```python
from build123d import *

# Parameters (mm, degrees)
BOSS_EXTRUDE2_DEPTH = 5


with BuildPart() as part:
    # Sketch3 → Boss-Extrude2 (new body)
    with BuildSketch(Plane(origin=(0, 0, 0), x_dir=(1, 0, 0), z_dir=(0, 1, 0))):
        with BuildLine():
            ThreePointArc((-2.946687169, 0.278195868), (-2.823196953, -0.888772849), (-2.255920315, -1.916032813))
            add(Edge.make_bspline(
                [(-2.255920315, -1.916032813), (-13.171337356, -14.504845087), (-19.982146303, -0.549733438)],
                knots=[0, 0, 0, 1, 1, 1], degree=2))
            ThreePointArc((-19.982146303, -0.549733438), (-17.317507753, -9.984603294), (-10.487312447, -17.017774689))
            add(Edge.make_bspline(
                [(-1.000187104, -2.785674778), (-2.546841566, -12.490182628), (-10.487312447, -17.017774689)],
                knots=[0, 0, 0, 1, 1, 1], degree=2))
            ThreePointArc((-1.000187104, -2.785674778), (0.084052871, -2.958596513), (1.156726663, -2.724397481))
            add(Edge.make_bspline(
                [(1.156726663, -2.724397481), (13.351165317, -11.711219241), (1.815860807, -19.907059734)],
                knots=[0, 0, 0, 1, 1, 1], degree=2))
            ThreePointArc((1.815860807, -19.907059734), (9.30002387, -17.694573568), (15.366618382, -12.784968409))
            add(Edge.make_bspline(
                [(2.913240883, -0.522863047), (17.317700847, -1.946688078), (15.366618382, -12.784968409)],
                knots=[0, 0, 0, 1, 1, 1], degree=2))
            ThreePointArc((2.913240883, -0.522863047), (2.939564994, 0.345421275), (2.712677202, 1.183951269))
            add(Edge.make_bspline(
                [(2.712677202, 1.183951269), (12.295659798, 10.008861874), (19.989706794, 0)],
                knots=[0, 0, 0, 1, 1, 1], degree=2))
            ThreePointArc((19.989706794, 0), (18.426097238, 7.750310851), (13.979881947, 14.288151681))
            add(Edge.make_bspline(
                [(0, 2.959790231), (2.474515592, 15.075911373), (13.979881947, 14.288151681)],
                knots=[0, 0, 0, 1, 1, 1], degree=2))
            ThreePointArc((0, 2.959790231), (-1.229068634, 2.692535702), (-2.236179538, 1.939035658))
            add(Edge.make_bspline(
                [(-2.236179538, 1.939035658), (-13.359480088, 10.340651394), (-7.448796697, 18.550035189)],
                knots=[0, 0, 0, 1, 1, 1], degree=2))
            ThreePointArc((-7.448796697, 18.550035189), (-12.533274778, 15.572584919), (-16.528834056, 11.242153818))
            add(Edge.make_bspline(
                [(-2.946687169, 0.278195868), (-19.130769908, -2.126973155), (-16.528834056, 11.242153818)],
                knots=[0, 0, 0, 1, 1, 1], degree=2))
        make_face()
    extrude(amount=BOSS_EXTRUDE2_DEPTH)


solid = part.part
```
Work out the finished part from the listing and answer in its coordinate system (mm). A direction names the side the tool comes from. Coordinates: 2 decimals unless noted, no trailing zeros. Answer as CSV lines item,"result".
Q1. The part is cut by section A-A on x = -9. State how many separate pieces and enclosed holes the cut face has, and give its area (3 significant figures).
Findings:
separate pieces,"3"
enclosed holes,"0"
area,"105 mm²"
Q2. A tool of negligible diameter and unlimited length cuts with its end or side. For faces 4 (the face through (0, 0, 0)), 5 (the face through (-1.21, 2.46, -2.7)), from which of +Z, -Z, +X, -X, +Y, -Y can it reach the whole face along a straight path? Write none if from no direction.
Findings:
face 4,"+Z, -Z, +X, -X, -Y"
face 5,"-Z, +Y, -Y"
Q3. Find the intervals of material crossed by probe 1 along X at (y, z) = (1.95, -3); probe 2 along Z at (x, y) = (4.5, 4.3); probe 3 along X at (y, z) = (2.05, 5) (3 decimals), in increasing order.
Findings:
probe 1,"x = -15.55 to -3.57, 0.01 to 4.94, 17.15 to 19.76"
probe 2,"z = -11.66 to -2.68, 0.72 to 5.63, 17.68 to 19.48"
probe 3,"x = -19.354 to -17.155, -5.325 to -1.453, 3.877 to 13.862"
Q4. For a pull along Z with two mould halves and no side action, classify faces 1 (the face through (0, 5, 0)), 2 (the face through (-2.83, 2.46, 0.87)), 3 (the face through (-12.5, 2.5, -15.6)) as +Z half, -Z half, draft (parallel to the pull), parting line (faces both ways), or undercut.
Findings:
face 1,"draft"
face 2,"undercut"
face 3,"-Z half"
Q5. Each of these flat-tipped pins is pushed along its axis until it touches: pin 1 (2 mm diameter, centred on x = -8.5, y = 0.5, fed in from +Z); pin 2 (1 mm diameter, centred on y = 2, z = 5.5, fed in from +X); pin 3 (2 mm diameter, centred on x = 5, z = -5.5, fed in from -Y). Where does it stop, or does it pass through?
Findings:
pin 1,"stops at z = 16.42"
pin 2,"stops at x = 14.54"
pin 3,"stops at y = 0"
